```python
from build123d import *

# Parameters (mm, degrees)
SKETCH1_R           = 2.5
SKETCH1_W           = 6
SKETCH1_H           = 3
BOSS_EXTRUDE1_DEPTH = 6


with BuildPart() as part:
    # Sketch1 → Boss-Extrude1 (new body)
    with BuildSketch(Plane(origin=(0, 0, 0), x_dir=(1, 0, 0), z_dir=(0, 1, 0))):
        with BuildLine():
            Line((-6, 0), (-6, -25))
            Line((-6, -25), (-4, -25))
            Line((-4, -25), (-4, -31))
            Line((-4, -31), (4, -31))
            Line((4, -31), (4, -25))
            Line((4, -25), (6, -25))
            Line((6, -25), (6, 0))
            ThreePointArc((6, 0), (0, 6), (-6, 0))
        make_face()
        with Locations(Location((0, 0, 0), (0, 0, 270))):
            Circle(SKETCH1_R, mode=Mode.SUBTRACT)
        with Locations((0, -17.5)):
            Rectangle(SKETCH1_W, SKETCH1_H, mode=Mode.SUBTRACT)
    extrude(amount=BOSS_EXTRUDE1_DEPTH)


solid = part.part
```
Here's how the part is built. I have some questions about the finished solid (model axes, mm). A direction names the side the tool comes from. Coordinates: 2 decimals unless noted, no trailing zeros. Order: outer loops, then holes, each group sorted by start corner. A loop starts at its lowest first (then second) coordinate and runs counter-clockwise, first axis right, second up.
1) Which directions (+Z, -Z, +X, -X, +Y, -Y) give clear straight access to the entire face, cutting with the end or side of a thin tool? Please do faces 1 (the face through (6, 3, 13)), 2 (the face through (0, 3, 16)), 3 (the face through (-5, 3, 25)).
2) Imagine slicing it at D-D on x = -1.5. List the corners of the cut face in (y, z) for me, and give its area (3 significant figures).
3) Imagine slicing it at B-B on x = 0. List the corners of the cut face in (y, z) for me, and give its area (3 significant figures).
4) We'd pull the mould along X, two halves only. Please class faces 4 (the face through (0, 3, 19)), 5 (the face through (5, 3, 25)), 6 (the face through (0, 3, -6)), 7 (the face through (4, 3, 28)): +X half, -X half, draft (parallel to the pull), parting line (faces both ways), or undercut.
5) Imagine slicing it at A-A on z = 18.5. List the corners of the cut face in (x, y) for me.
6) Imagine slicing it at C-C on y = 4.8. List the corners of the cut face in (x, z) for me.
7) I need wall thicknesses on line 1 (X direction, y = 3.8, z = 0); line 2 (Z direction, x = -1.5, y = 4.2); line 3 (Z direction, x = 0.5, y = 0.75). Which ranges of each line are inside material? Lowest first, please.
8) Will this pin go through, and if not, where does the flat tip stop? pin 1 (2 mm diameter, centred on x = -5.5, y = 3, fed in from +Z).
Response values:
1. face 1: +Z, -Z, +X, +Y, -Y
1. face 2: +Y, -Y
1. face 3: +Z, -X, +Y, -Y
2. outline: (0, -5.81) - (6, -5.81) - (6, -2) - (0, -2) - close; (0, 2) - (6, 2) - (6, 16) - (0, 16) - close; (0, 19) - (6, 19) - (6, 31) - (0, 31) - close
2. area: 179 mm2
3. outline: (0, -6) - (6, -6) - (6, -2.5) - (0, -2.5) - close; (0, 2.5) - (6, 2.5) - (6, 16) - (0, 16) - close; (0, 19) - (6, 19) - (6, 31) - (0, 31) - close
3. area: 174 mm2
4. face 4: undercut
4. face 5: draft
4. face 6: parting line
4. face 7: +X half
5. outline: (-6, 0) - (-3, 0) - (-3, 6) - (-6, 6) - close; (3, 0) - (6, 0) - (6, 6) - (3, 6) - close
6. outline: (-6, 0) arc R6 ccw to (6, 0) - (6, 25) - (4, 25) - (4, 31) - (-4, 31) - (-4, 25) - (-6, 25) - close; hole (-3, 16) - (3, 16) - (3, 19) - (-3, 19) - close; hole circle Ø5 at (0, 0)
7. line 1: x = -6 to -2.5, 2.5 to 6
7. line 2: z = -5.81 to -2, 2 to 16, 19 to 31
7. line 3: z = -5.98 to -2.45, 2.45 to 16, 19 to 31
8. pin 1: stops at z = 25
